Input: part model. Units: mm. Frame: model coordinates. Face numbers are marked on the shaded views. A direction names the side the tool comes from. Give positions to 0.01 mm unless a question says otherwise; leave off trailing zeros. Loops run counter-clockwise (first coordinate to the right, second up) from the corner with the lowest first, then second, coordinate; pieces in that order, holes last. Notation, with made-up numbers: M 89.25,23 L 148.25,23 A18 cw 148.25,37 Z; hole C -6.5,25.5 d6. An arc over 180 degrees is marked long. Use CSV: the item, a comma, the result in double quotes. Start each with the question number.
Q1. Section B-B, the plane y = -291.5. Output: boundary loops of the cut face in (x, z), plus the area to 3 significant figures.
Q2. Section C-C, the plane z = 33.5. Output: boundary loops of the cut face in (x, y), plus the area to 4 significant figures.
Q3. Pin query (flat end, axial travel): pin 1 (6 mm diameter, centred on x = 125, y = -79.5, fed in from -Z); pin 2 (10 mm diameter, centred on x = -398.5, y = -129, fed in from +Z). Return the tip coordinate at first contact, or that it passes through.
Q4. Material intervals for line 1 along Y through (x, z) = (-321, -18); line 2 along X through (y, z) = (341, -72); line 3 along X through (y, z) = (-297, 21), sorted ascending.
Q5. Pull-direction query (X, two-part tool) for the marked faces 4, 5, 6 and 7; classes: released by +X, released by -X, zero draft, split by the parting line, or undercut.
Q6. Section A-A, the plane x = 471.5. Output: boundary loops of the cut face in (y, z).
Q7. Reachability of the marked faces 1, 2 and 3 from +Z, -Z, +X, -X, +Y, -Y: full face, straight path, thin tool, end or side. Return the list, or none.
from build123d import *

# Parameters (mm, degrees)
F0_W     = 1500
F0_H     = 1000
F0_W_2   = 675
F0_H_2   = 425
F1_DEPTH = 125
F2_W     = 675
F2_H     = 425
F3_DEPTH = 3


with BuildPart() as f1:
    # F0 (on Top) → F1 (new body, symmetric)
    with BuildSketch(Plane.XY):
        Rectangle(F0_W, F0_H)
        with Locations((-372.967375, -237.5)):
            Rectangle(F0_W_2, F0_H_2, mode=Mode.SUBTRACT)
        with Locations((362.5, -237.5)):
            Rectangle(F0_W_2, F0_H_2, mode=Mode.SUBTRACT)
        with Locations((-364.561057, 237.5)):
            Rectangle(F0_W_2, F0_H_2, mode=Mode.SUBTRACT)
        with Locations((360.438943, 237.5)):
            Rectangle(F0_W_2, F0_H_2, mode=Mode.SUBTRACT)
    extrude(amount=F1_DEPTH, both=True)

    # F2 (on Top) → F3 (join)
    with BuildSketch(Plane.XY):
        with Locations((-368.367167, 242.65543)):
            Rectangle(F2_W, F2_H)
        with Locations((-368.367167, -233.154571)):
            Rectangle(F2_W, F2_H)
        with Locations((359.504882, 242.65543)):
            Rectangle(F2_W, F2_H)
        with Locations((359.504882, -237.751758)):
            Rectangle(F2_W, F2_H)
    extrude(amount=F3_DEPTH)


solid = f1.part
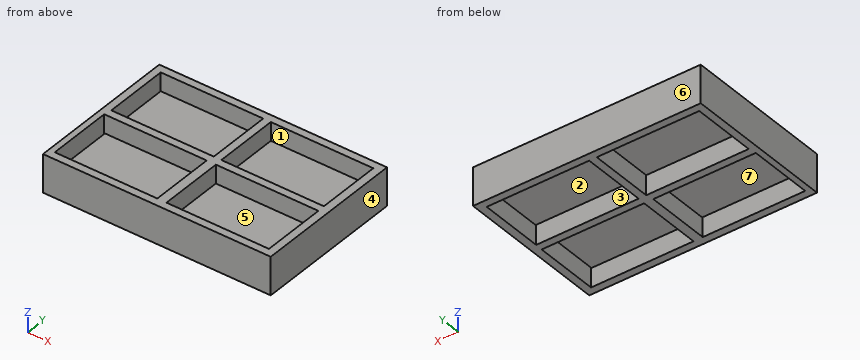
A:
1,outline,"M -750,-125 L -710.47,-125 L -710.47,125 L -750,125 Z; M -705.87,0 L -35.47,0 L -35.47,-125 L 25,-125 L 25,0 L 697,0 L 697,3 L 25,3 L 25,125 L -35.47,125 L -35.47,3 L -705.87,3 Z; M 700,-125 L 750,-125 L 750,125 L 700,125 Z"
1,area,"41,500 mm^2"
2,outline,"M -750,-500 L 750,-500 L 750,500 L -750,500 Z; hole M -710.47,-450 L -35.47,-450 L -35.47,-25 L -710.47,-25 Z; hole M -702.06,25 L -27.06,25 L -27.06,450 L -702.06,450 Z; hole M 22.94,25 L 697.94,25 L 697.94,450 L 22.94,450 Z; hole M 25,-450 L 700,-450 L 700,-25 L 25,-25 Z"
2,area,"352,500 mm^2"
3,pin 1,"z = 0"
3,pin 2,"z = 3"
4,line 1,"-500 to -450, -25 to 25, 450 to 500"
4,line 2,"-750 to -702.06, -27.06 to 22.94, 697.94 to 750"
4,line 3,"-750 to -710.47, -35.47 to 25, 700 to 750"
5,face 4,"released by +X"
5,face 5,"undercut"
5,face 6,"zero draft"
5,face 7,"undercut"
6,outline,"M -500,-125 L -450,-125 L -450,0 L -25.25,0 L -25.25,3 L -450,3 L -450,125 L -500,125 Z; M -25,-125 L 25,-125 L 25,125 L -25,125 Z; M 30.16,0 L 450,0 L 450,-125 L 500,-125 L 500,125 L 450,125 L 450,3 L 30.16,3 Z"
7,face 1,"none"
7,face 2,"-Z"
7,face 3,"+Z, -Z"
